The listing builds one solid part. Answer for the finished solid, in the listing's coordinates (mm). A direction names the side the tool comes from. Round coordinates to 2 decimals unless told otherwise and drop trailing zeros. Loops run counter-clockwise (first coordinate to the right, second up) from the corner with the lowest first, then second, coordinate; pieces in that order, holes last. Notation, with made-up numbers: (20, 89.5) -> (72, 89.5) arc R23 cw to (72, 114.5) -> close; hole circle Ø5 at (40, 73.5). An arc over 180 degrees is marked (long way). Use a Markdown table: item, result. Add a question column.
Q1. Section A-A on x = 5.5 is taken. Give the vertices of the cut face in (y, z), then the cut area to 3 significant figures.
Q2. For a pull along X with two mould halves and no side action, classify faces 1 (the cylindrical face through (28.14, 8.86, 9.86)), 2 (the flat face through (0, 0, 0)), 3 (the cylindrical face through (13.912, 20.772, 0.493)), 4 (the flat face through (-6.33, -12.7, 0.49)) as released by +X, released by -X, zero draft, split by the parting line, or undercut.
Q3. Which of the six approach directions +Z, -Z, +X, -X, +Y, -Y give full straight-line access (tool end or side, diameter ignored) to faces 5 (the flat face through (-7.835, 11.834, 0.493)), 6 (the cylindrical face through (26.327, -10.916, 10.367)), 7 (the flat face through (-15.4, 24.2, 20))?
Q4. Given pin 1 Ø3 at (x, z) = (-19, 11.5) entering from +Y; pin 2 Ø1.5 at (x, y) = (-0.5, -0.5) entering from +Z; pin 3 Ø4 at (x, z) = (6.5, 15.5) entering from +Y, each flat-ended and moving along its own axis, determine where each tip first touches the part or whether it passes through.
Q5. Section C-C on z = 2.25 is taken. Give the vertices of the cut face in (x, y), then the cut area to 3 significant figures.
Q6. Section D-D on z = 18.25 is taken. Give the vertices of the cut face in (x, y), then the cut area to 3 significant figures.
Q7. Section B-B on y = -11.5 is taken. Give the vertices of the cut face in (x, z).
Q8. Consider line 1 (Y direction, x = 0, z = 15.25); line 2 (Y direction, x = 17, z = 7.25); line 3 (X direction, y = -9, z = 17). Determine where each line is inside the solid, lowest interval first.
from build123d import *

# Parameters (mm, degrees)
F0_R     = 29.5
F0_R_2   = 28.5
F1_DEPTH = 20
F2_DEPTH = 1
F3_R     = 1.5
F4_DEPTH = 3


with BuildPart() as f1:
    # F0 (on Top) → F1 (new body)
    with BuildSketch(Plane.XY):
        Circle(F0_R)
        Circle(F0_R_2, mode=Mode.SUBTRACT)
    extrude(amount=F1_DEPTH)

    # F0 (on Top) → F2 (join)
    with BuildSketch(Plane.XY):
        Circle(F0_R_2)
        with BuildLine():
            ThreePointArc((-8.887001, 23.367097), (14.191987, 20.581242), (25, 0))
            ThreePointArc((25, 0), (24.919872, -2), (24.68, -3.987179))
            ThreePointArc((24.68, -3.987179), (10.727885, -22.581242), (-12.5, -21.650635))
            ThreePointArc((-12.5, -21.650635), (-14.191987, -20.581242), (-15.792999, -19.379917))
            ThreePointArc((-15.792999, -19.379917), (-24.919872, 2), (-12.5, 21.650635))
            ThreePointArc((-12.5, 21.650635), (-10.727885, 22.581242), (-8.887001, 23.367097))
        make_face(mode=Mode.SUBTRACT)
        with BuildLine():
            Line((0.575662, 3.452335), (-8.887001, 23.367097))
            ThreePointArc((-8.887001, 23.367097), (-10.727885, 22.581242), (-12.5, 21.650635))
            Line((-12.5, 21.650635), (-3.038183, 1.737654))
            ThreePointArc((-3.038183, 1.737654), (-1.500345, 3.162114), (0.575662, 3.452335))
        make_face()
        with BuildLine():
            ThreePointArc((-15.792999, -19.379917), (-14.191987, -20.581242), (-12.5, -21.650635))
            Line((-12.5, -21.650635), (0.014239, -3.499971))
            ThreePointArc((0.014239, -3.499971), (-1.988299, -2.880394), (-3.27764, -1.22763))
            Line((-3.27764, -1.22763), (-15.792999, -19.379917))
        make_face()
        with BuildLine():
            ThreePointArc((3.5, 0), (3.378891, 0.912742), (3.023944, 1.762317))
            ThreePointArc((3.023944, 1.762317), (1.988299, 2.880394), (0.575662, 3.452335))
            ThreePointArc((0.575662, 3.452335), (-1.500345, 3.162114), (-3.038183, 1.737654))
            ThreePointArc((-3.038183, 1.737654), (-3.488644, 0.28172), (-3.27764, -1.22763))
            ThreePointArc((-3.27764, -1.22763), (-1.988299, -2.880394), (0.014239, -3.499971))
            ThreePointArc((0.014239, -3.499971), (1.500345, -3.162114), (2.701978, -2.224705))
            ThreePointArc((2.701978, -2.224705), (3.294459, -1.181752), (3.5, 0))
        make_face()
        with BuildLine():
            ThreePointArc((24.68, -3.987179), (24.919872, -2), (25, 0))
            Line((25, 0), (3.023944, 1.762317))
            ThreePointArc((3.023944, 1.762317), (3.378891, 0.912742), (3.5, 0))
            ThreePointArc((3.5, 0), (3.294459, -1.181752), (2.701978, -2.224705))
            Line((2.701978, -2.224705), (24.68, -3.987179))
        make_face()
    extrude(amount=F2_DEPTH)

    # F3 (on face) → F4 (join)
    with BuildSketch(Plane.XY.offset(1)):
        Circle(F3_R)
    extrude(amount=F4_DEPTH)


solid = f1.part
Checked values:
| question | item | result |
|---|---|---|
| 1 | outline | (-28.98, 0) -> (-24.39, 0) -> (-24.39, 1) -> (-27.96, 1) -> (-27.96, 20) -> (-28.98, 20) -> close; (-2.45, 0) -> (1.56, 0) -> (1.56, 1) -> (-2.45, 1) -> close; (24.39, 0) -> (28.98, 0) -> (28.98, 20) -> (27.96, 20) -> (27.96, 1) -> (24.39, 1) -> close |
| 1 | area | 51.9 mm2 |
| 2 | face 1 | split by the parting line |
| 2 | face 2 | zero draft |
| 2 | face 3 | undercut |
| 2 | face 4 | undercut |
| 3 | face 5 | +Z, -Z |
| 3 | face 6 | +Z |
| 3 | face 7 | +Z, +X, -X, +Y, -Y |
| 4 | pin 1 | stops at y = 23.75 |
| 4 | pin 2 | stops at z = 4 |
| 4 | pin 3 | stops at y = 29.15 |
| 5 | outline | circle Ø59 at (0, 0); circle Ø3 at (0, 0); hole circle Ø57 at (0, 0) |
| 5 | area | 189 mm2 |
| 6 | outline | circle Ø59 at (0, 0); hole circle Ø57 at (0, 0) |
| 6 | area | 182 mm2 |
| 7 | outline | (-27.17, 0) -> (-22.2, 0) -> (-22.2, 1) -> (-26.08, 1) -> (-26.08, 20) -> (-27.17, 20) -> close; (-10.36, 0) -> (-5.5, 0) -> (-5.5, 1) -> (-10.36, 1) -> close; (22.2, 0) -> (27.17, 0) -> (27.17, 20) -> (26.08, 20) -> (26.08, 1) -> (22.2, 1) -> close |
| 8 | line 1 | y = -29.5 to -28.5, 28.5 to 29.5 |
| 8 | line 2 | y = -24.11 to -22.87, 22.87 to 24.11 |
| 8 | line 3 | x = -28.09 to -27.04, 27.04 to 28.09 |
